Drawing for the job (mm, zero at the part's lowest x, y, z). A direction names the side the tool comes from. Give positions to 0.01 mm unless a question says otherwise; leave off trailing zeros. Order: outer loops, then holes, each group sorted by start corner. A loop starts at its lowest first (then second) coordinate and runs counter-clockwise, first axis right, second up. Notation, with made-up numbers: M 54,-33.75 L 80,-33.75 A8 ccw 80,-21.75 Z; hole C 23.5,-14 d1. An arc over 180 degrees is marked long. One line per item, written item: value.
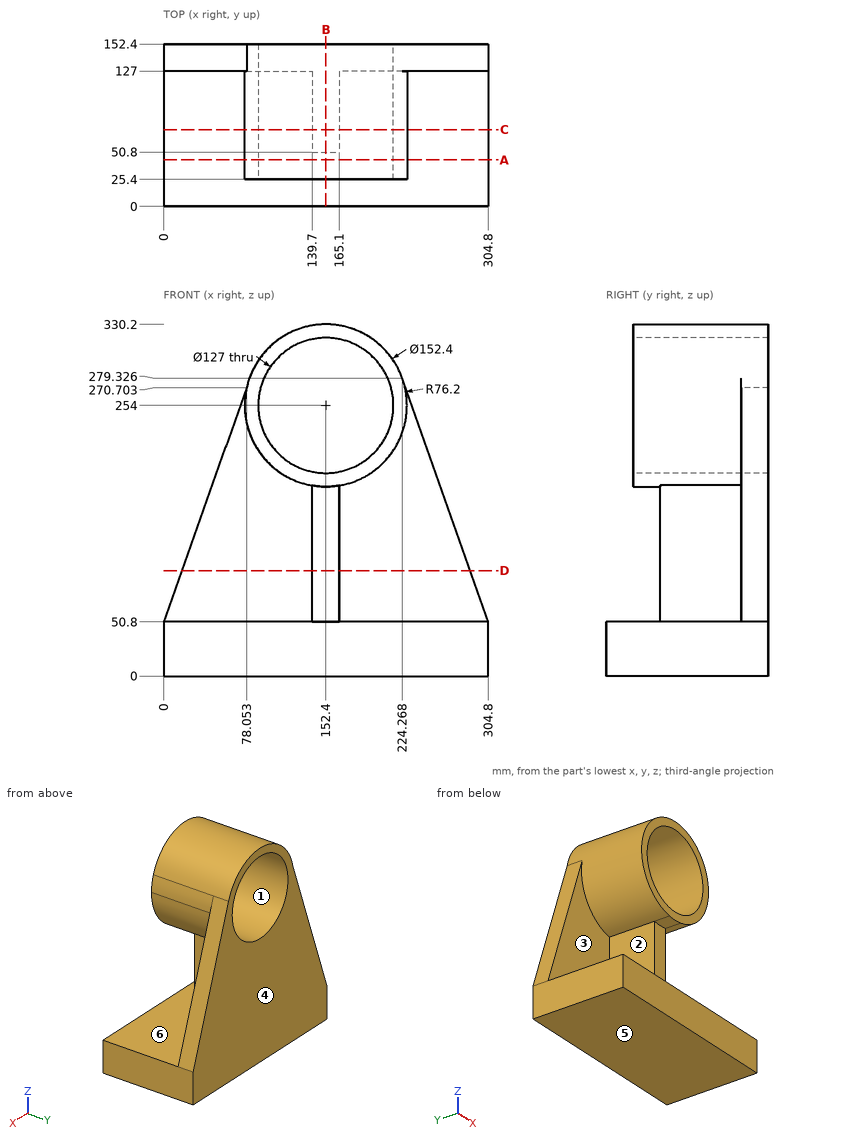
1) Saw through at C-C, the plane y = 72. Write the cut outline in (x, z), then the cut area to 3 significant figures.
Check values:
outline: M 0,0 L 304.8,0 L 304.8,50.8 L 165.1,50.8 L 165.1,178.87 A76.2 ccw long 139.7,178.87 L 139.7,50.8 L 0,50.8 Z; hole C 152.4,254 d127
area: 24,300 mm^2
2) Mould opens along Z. For the marked faces 3, 4, 5 and 6 say: released by +Z, released by -Z, zero draft, split by the parting line, or undercut.
Check values:
face 3: undercut
face 4: zero draft
face 5: released by -Z
face 6: undercut
3) Saw through at B-B, the plane x = 152.4. Write the cut outline in (y, z), then the cut area to 3 significant figures.
Check values:
outline: M 0,0 L 152.4,0 L 152.4,190.5 L 25.4,190.5 L 25.4,177.8 L 50.8,177.8 L 50.8,50.8 L 0,50.8 Z; M 25.4,317.5 L 152.4,317.5 L 152.4,330.2 L 25.4,330.2 Z
area: 23,900 mm^2
4) Pin check, flat tips, straight feed: pin 1 (8 mm diameter, centred on x = 86, y = 112, fed in from +Z) (1 decimal); pin 2 (10 mm diameter, centred on y = 116, z = 220, fed in from +X); pin 3 (7.5 mm diameter, centred on x = 158.5, z = 96, fed in from -Y). Stop position of each tip, or through.
Check values:
pin 1: z = 297.7
pin 2: x = 222.87
pin 3: y = 50.8
5) Drill centre lines: probe 1 along Z at (x, y) = (152.4, 109); probe 2 along Z at (x, y) = (196, 103) (1 decimal); probe 3 along Y at (x, z) = (74.5, 90.5). Where is each one in solid material? Low to high. Write a range as from..to.
Check values:
probe 1: 0..190.5, 317.5..330.2
probe 2: 0..50.8, 191.5..207.8, 300.2..316.5
probe 3: 127..152.4
6) Saw through at A-A, the plane y = 43.5. Write the cut outline in (x, z).
Check values:
outline: M 0,0 L 304.8,0 L 304.8,50.8 L 0,50.8 Z; C 152.4,254 d152.4; hole C 152.4,254 d127
7) Saw through at D-D, the plane z = 99. Write the cut outline in (x, y).
Check values:
outline: M 17.11,127 L 139.7,127 L 139.7,50.8 L 165.1,50.8 L 165.1,127 L 287.81,127 L 287.81,152.4 L 17.11,152.4 Z
8) Tool access for the marked faces 1 and 2: list every direction of +Z, -Z, +X, -X, +Y, -Y with a clear straight run to the whole face (end or side of a thin tool).
Check values:
face 1: +Y, -Y
face 2: -X, -Y
